```python
from build123d import *

# Parameters (mm, degrees)
BOSS_EXTRUDE1_DEPTH      = 2.5
SKETCH4_R                = 0.35
THROUGH_HOLES_DEPTH      = 4.688156721
FILLET1_R                = 0.125
BOSS_EXTRUDE4_DEPTH      = 0.5
BOSS_EXTRUDE4_DEPTH_BACK = 0.25
SKETCH11_W               = 4
SKETCH11_H               = 8.35
SKETCH12_W               = 0.4
SKETCH12_H               = 8.35
BOSS_EXTRUDE5_DEPTH      = 0.5


with BuildPart() as part:
    # Sketch3 → Boss-Extrude1 (new body)
    with BuildSketch(Plane(origin=(0, 0, 0), x_dir=(1, 0, 0), z_dir=(0, 1, 0))):
        with BuildLine():
            Line((-2.5, 0.9), (-2, 0.93))
            Line((-2, 0.93), (-2, 0.56))
            Line((-2, 0.56), (-1.5, 0.56))
            Line((-1.5, 0.56), (-1.5, 0.96))
            Line((-1.5, 0.96), (0, 1.05))
            ThreePointArc((0, 1.05), (1.05, 0), (0, -1.05))
            Line((0, -1.05), (-1.5, -0.96))
            Line((-1.5, -0.96), (-1.5, -0.56))
            Line((-1.5, -0.56), (-2, -0.56))
            Line((-2, -0.56), (-2, -0.93))
            Line((-2, -0.93), (-2.5, -0.9))
            Line((-2.5, -0.9), (-2.5, 0.9))
        make_face()
    extrude(amount=BOSS_EXTRUDE1_DEPTH)

    # Sketch4 → Through Holes (cut, through all)
    with BuildSketch(Plane(origin=(0, 2.5, 0), x_dir=(1, 0, 0), z_dir=(0, 1, 0))):
        with Locations(Location((0, 0, 0), (0, 0, 270))):
            Circle(SKETCH4_R)
    extrude(amount=-THROUGH_HOLES_DEPTH, mode=Mode.SUBTRACT)

    # Fillet1
    fillet1_edges = [part.edges().sort_by_distance(p)[0] for p in [
        (-2, 1.25, -0.56),
        (-1.5, 1.25, -0.56),
        (-1.5, 1.25, 0.56),
        (-2, 1.25, 0.56),
    ]]
    fillet(fillet1_edges, radius=FILLET1_R)

    # Sketch11 → Boss-Extrude4 (add, two sides: drawn at the far end of the back side and taken through both)
    with BuildSketch(Plane.ZY.offset(2.5).offset(-BOSS_EXTRUDE4_DEPTH_BACK)):
        with Locations((0, 0.325)):
            Rectangle(SKETCH11_W, SKETCH11_H)
    extrude(amount=BOSS_EXTRUDE4_DEPTH + BOSS_EXTRUDE4_DEPTH_BACK)

    # Sketch12 → Boss-Extrude5 (add)
    with BuildSketch(Plane.ZY.offset(3)):
        with Locations((-1.8, 0.325)):
            Rectangle(SKETCH12_W, SKETCH12_H)
    extrude(amount=BOSS_EXTRUDE5_DEPTH)


solid = part.part
```
Geometry: final body of the model. Coordinates: model frame, mm. A direction names the side the tool comes from. Coordinates: 2 decimals unless noted, no trailing zeros. Order: outer loops, then holes, each group sorted by start corner. A loop starts at its lowest first (then second) coordinate and runs counter-clockwise, first axis right, second up. Notation, with made-up numbers: (-2.5, 49) -> (31.5, 49) arc R14 cw to (31.5, 74) -> close; hole circle Ø3 at (-39.5, -38). An arc over 180 degrees is marked (long way). Answer in a Markdown table with one row per item.
Item 1: Draft query along X for faces 1 (the flat face through (-0.74, 1.232, 1.006)), 2 (the cylindrical face through (1.05, 1.23, -0.02)), 3 (the flat face through (-3, 0, 0)), 4 (the flat face through (-1, 2.5, 0)). Return one class per face: released by +X, released by -X, zero draft, split by the parting line, or undercut.
Return value:
| item | result |
|---|---|
| face 1 | undercut |
| face 2 | released by +X |
| face 3 | released by -X |
| face 4 | zero draft |
Item 2: Section A-A on y = 1.25. Output: boundary loops of the cut face in (x, z) (3 decimals), plus the area to 3 significant figures.
Return value:
| item | result |
|---|---|
| outline | (-3.5, -2) -> (-2.25, -2) -> (-2.25, -0.915) -> (-2, -0.93) -> (-2, -0.685) arc R0.125 cw to (-1.875, -0.56) -> (-1.625, -0.56) arc R0.125 cw to (-1.5, -0.685) -> (-1.5, -0.96) -> (0, -1.05) arc R1.05 ccw to (0, 1.05) -> (-1.5, 0.96) -> (-1.5, 0.685) arc R0.125 cw to (-1.625, 0.56) -> (-1.875, 0.56) arc R0.125 cw to (-2, 0.685) -> (-2, 0.93) -> (-2.25, 0.915) -> (-2.25, 2) -> (-3, 2) -> (-3, -1.6) -> (-3.5, -1.6) -> close; hole circle Ø0.7 at (0, 0) |
| area | 8.60 mm² |
Item 3: Ray query, L1, parallel to X at y = 0.95, z = 0; L2, parallel to Z at x = -1.6, y = 2.25; L3, parallel to Y at x = -0.9, z = 0.45. Return the intervals inside material, ascending.
Return value:
| item | result |
|---|---|
| L1 | x = -3 to -0.35, 0.35 to 1.05 |
| L2 | z = -0.56 to 0.56 |
| L3 | y = 0 to 2.5 |
Item 4: Contact query for flat-ended pins moving along their axis: P1, Ø2, axis at x = -1, z = 0, coming from the +Y side; P2, Ø1, axis at y = 2.5, z = -1, coming from the -X side. Output: stop coordinate, or through.
Return value:
| item | result |
|---|---|
| P1 | stops at y = 2.5 |
| P2 | stops at x = -3 |
Item 5: Section B-B on z = 0. Output: boundary loops of the cut face in (x, y), plus the area to 3 significant figures.
Return value:
| item | result |
|---|---|
| outline | (-3, -3.85) -> (-2.25, -3.85) -> (-2.25, 0) -> (-0.35, 0) -> (-0.35, 2.5) -> (-2.25, 2.5) -> (-2.25, 4.5) -> (-3, 4.5) -> close; (0.35, 0) -> (1.05, 0) -> (1.05, 2.5) -> (0.35, 2.5) -> close |
| area | 12.8 mm² |
Item 6: Access query for faces 5 (the flat face through (-1, 0, 0)), 6 (the flat face through (-2.6, -3.85, 0)), 7 (the flat face through (-0.8, 1.2, -1)). Directions: +Z, -Z, +X, -X, +Y, -Y. A direction counts if a zero-diameter tool reaches every point of the face in a straight line with its end or side. Return the directions, or none.
Return value:
| item | result |
|---|---|
| face 5 | +Z, -Z, +X, -Y |
| face 6 | +Z, -Z, +X, -X, -Y |
| face 7 | -Z, +Y, -Y |
Item 7: Section C-C on x = -0.25. Output: boundary loops of the cut face in (y, z) (3 decimals), plus the area to 3 significant figures.
Return value:
| item | result |
|---|---|
| outline | (0, -1.035) -> (2.5, -1.035) -> (2.5, -0.245) -> (0, -0.245) -> close; (0, 0.245) -> (2.5, 0.245) -> (2.5, 1.035) -> (0, 1.035) -> close |
| area | 3.95 mm² |
Item 8: Section D-D on y = 3. Output: boundary loops of the cut face in (x, z), plus the area to 3 significant figures.
Return value:
| item | result |
|---|---|
| outline | (-3.5, -2) -> (-2.25, -2) -> (-2.25, 2) -> (-3, 2) -> (-3, -1.6) -> (-3.5, -1.6) -> close |
| area | 3.20 mm² |
